```python
from build123d import *

# Parameters (mm, degrees)
SKETCH_1_R             = 18.5
EXTRUDE_1_DEPTH        = 26.5
SKETCH_2_R             = 6
EXTRUDE_2_DEPTH        = 6
SKETCH_3_R             = 3
EXTRUDE_3_DEPTH        = 15.5
SKETCH_4_W             = 6.445073496
SKETCH_4_H             = 1.792044826
CUT_EXTRUDE_1_DEPTH    = 12
SKETCH_5_R             = 16.5
EXTRUDE_4_DEPTH        = 22
HOLE_WIZARD_M3_1_D     = 2.5
HOLE_WIZARD_M3_1_DEPTH = 7.5
HOLE_WIZARD_M3_1_TIP   = 0.751075774
SKETCH_8_R             = 14
EXTRUDE_5_DEPTH        = 4.5
CUT_EXTRUDE_START      = -2.5
SKETCH_9_R             = 14
SKETCH_9_R_2           = 8
CUT_EXTRUDE_2_DEPTH    = 2.5
CUT_EXTRUDE_START_2    = -3
SKETCH_10_R            = 14
SKETCH_10_R_2          = 9.657403228
CUT_EXTRUDE_3_DEPTH    = 3


with BuildPart() as part:
    # 草图1 → 凸台-拉伸1 (new body)
    with BuildSketch(Plane.XY):
        Circle(SKETCH_1_R)
    extrude(amount=EXTRUDE_1_DEPTH)

    # 草图2 → 凸台-拉伸2 (add)
    with BuildSketch(Plane.XY.offset(26.5)):
        with Locations((0, 7)):
            Circle(SKETCH_2_R)
    extrude(amount=EXTRUDE_2_DEPTH)

    # 草图3 → 凸台-拉伸3 (add)
    with BuildSketch(Plane.XY.offset(32.5)):
        with Locations((0, 7)):
            Circle(SKETCH_3_R)
    extrude(amount=EXTRUDE_3_DEPTH)

    # 草图4 → 切除-拉伸1 (cut)
    with BuildSketch(Plane.XY.offset(48)):
        with Locations((0.299511506, 10.296022413)):
            Rectangle(SKETCH_4_W, SKETCH_4_H)
    extrude(amount=-CUT_EXTRUDE_1_DEPTH, mode=Mode.SUBTRACT)

    # 草图5 → 凸台-拉伸4 (add)
    with BuildSketch(Plane(origin=(0, 0, 0), x_dir=(-1, 0, 0), z_dir=(0, 0, -1))):
        with Locations(Location((0, 0, 0), (0, 0, 180))):
            Circle(SKETCH_5_R)
    extrude(amount=EXTRUDE_4_DEPTH)

    # M3 螺纹孔1
    with Locations(Plane(origin=(-7.75, 13.423393759, 26.5), x_dir=(1, 0, 0), z_dir=(0, 0, 1))):
        with Locations((0, 0), (15.5, 0), (23.25, -13.423393759), (15.5, -26.846787518), (0, -26.846787518), (-7.75, -13.423393759)):
            Hole(HOLE_WIZARD_M3_1_D / 2, depth=HOLE_WIZARD_M3_1_DEPTH)
            with Locations((0, 0, -(HOLE_WIZARD_M3_1_DEPTH + HOLE_WIZARD_M3_1_TIP / 2))):  # 118° drill point
                Cone(0, HOLE_WIZARD_M3_1_D / 2, HOLE_WIZARD_M3_1_TIP, mode=Mode.SUBTRACT)

    # 草图8 → 凸台-拉伸5 (add)
    with BuildSketch(Plane(origin=(0, 0, -22), x_dir=(-1, 0, 0), z_dir=(0, 0, -1))):
        Circle(SKETCH_8_R)
    extrude(amount=EXTRUDE_5_DEPTH)

    # 草图9 → 切除-拉伸2 (cut)
    with BuildSketch(Plane(origin=(0, 0, -24.5), x_dir=(-1, 0, 0), z_dir=(0, 0, -1)).offset(CUT_EXTRUDE_START)):
        Circle(SKETCH_9_R)
        Circle(SKETCH_9_R_2, mode=Mode.SUBTRACT)
    extrude(amount=CUT_EXTRUDE_2_DEPTH, mode=Mode.SUBTRACT)

    # 草图10 → 切除-拉伸3 (cut)
    with BuildSketch(Plane(origin=(0, 0, -26.5), x_dir=(-1, 0, 0), z_dir=(0, 0, -1)).offset(CUT_EXTRUDE_START_2)):
        Circle(SKETCH_10_R)
        Circle(SKETCH_10_R_2, mode=Mode.SUBTRACT)
    extrude(amount=CUT_EXTRUDE_3_DEPTH, mode=Mode.SUBTRACT)


solid = part.part
```
Could you check a few things on this model? Use its own coordinates, in mm. A direction names the side the tool comes from. Round coordinates to 2 decimals unless told otherwise and drop trailing zeros. Loops run counter-clockwise (first coordinate to the right, second up) from the corner with the lowest first, then second, coordinate; pieces in that order, holes last. Notation, with made-up numbers: M 20,38.25 L 43,38.25 A16 ccw 43,43.25 Z; hole C 60,-31 d2. An arc over 180 degrees is marked long. Put each result on its own line as item: value.
Q1. For pin 1 (3 mm diameter, centred on x = 7.75, y = -13.42, fed in from +Z); pin 2 (1.5 mm diameter, centred on x = -6.5, y = 7, fed in from +Z); pin 3 (2 mm diameter, centred on x = 7.75, y = 13.42, fed in from -Z), each with a flat end and sliding along its axis, tell me the tip position at first contact or that it passes through.
Check result:
pin 1: z = 26.5
pin 2: z = 32.5
pin 3: z = -22
Q2. Imagine slicing it at C-C (z = 38). Write out the boundary of the cut face in (x, y).
Check result:
outline: M -1.8,9.4 A3 ccw long 1.8,9.4 Z
Q3. I need wall thicknesses on probe 1 along Z at (x, y) = (7, 5); probe 2 along Y at (x, z) = (7, 25); probe 3 along Y at (x, z) = (7.75, 24). Which ranges of each line are inside material? Lowest first, please.
Check result:
probe 1: -26.5 to -24.5, -22 to 26.5
probe 2: -17.12 to -14.42, -12.42 to 12.42, 14.42 to 17.12
probe 3: -16.8 to -14.67, -12.17 to 12.17, 14.67 to 16.8
Q4. Imagine slicing it at D-D (y = -7). Write out the boundary of the cut face in (x, z).
Check result:
outline: M -17.12,0 L -14.94,0 L -14.94,-22 L -3.87,-22 L -3.87,-24.5 L -6.65,-24.5 L -6.65,-26.5 L 6.65,-26.5 L 6.65,-24.5 L 3.87,-24.5 L 3.87,-22 L 14.94,-22 L 14.94,0 L 17.12,0 L 17.12,26.5 L -17.12,26.5 Z
Q5. Thinking about a two-plate mould opening in X: for faces 6 (the face through (-4.01, -18.06, 13.06)), 7 (the face through (7.59, -13.28, 18.38)), 8 (the face through (-17, 0, 0)), which applies, released by +X, released by -X, zero draft, split by the parting line, or undercut?
Check result:
face 6: split by the parting line
face 7: undercut
face 8: zero draft
Q6. Imagine slicing it at A-A (x = 0). Write out the boundary of the cut face in (y, z), then the cut area to 3 significant figures.
Check result:
outline: M -18.5,0 L -16.5,0 L -16.5,-22 L -8,-22 L -8,-24.5 L -9.66,-24.5 L -9.66,-26.5 L 9.66,-26.5 L 9.66,-24.5 L 8,-24.5 L 8,-22 L 16.5,-22 L 16.5,0 L 18.5,0 L 18.5,26.5 L 13,26.5 L 13,32.5 L 10,32.5 L 10,36 L 9.4,36 L 9.4,48 L 4,48 L 4,32.5 L 1,32.5 L 1,26.5 L -18.5,26.5 Z
area: 1,940 mm2
Q7. Imagine slicing it at B-B (y = 7). Write out the boundary of the cut face in (x, z), then the cut area to 3 significant figures.
Check result:
outline: M -17.12,0 L -14.94,0 L -14.94,-22 L -3.87,-22 L -3.87,-24.5 L -6.65,-24.5 L -6.65,-26.5 L 6.65,-26.5 L 6.65,-24.5 L 3.87,-24.5 L 3.87,-22 L 14.94,-22 L 14.94,0 L 17.12,0 L 17.12,26.5 L 6,26.5 L 6,32.5 L 3,32.5 L 3,48 L -3,48 L -3,32.5 L -6,32.5 L -6,26.5 L -17.12,26.5 Z
area: 1,780 mm2
Q8. On a 3-axis mill with a long thin cutter (end or side, diameter ignored), from which of +Z, -Z, +X, -X, +Y, -Y can I reach the whole of each face in a straight line? I mean faces 1 (the face through (-9.21, 2.9, -25.49)), 2 (the face through (0, 9.4, 42)), 3 (the face through (0, 0, -26.5)), 4 (the face through (16.75, 0.05, 22.7)), 5 (the face through (0, 7, 48)). Say none if no direction works.
Check result:
face 1: -Z
face 2: +Z, +X, -X, +Y
face 3: -Z, +X, -X, +Y, -Y
face 4: +Z
face 5: +Z, +X, -X, +Y, -Y
